from build123d import *

# Parameters (mm, degrees)
SKETCH1_W           = 279.4
SKETCH1_H           = 254
BOSS_EXTRUDE1_DEPTH = 4.800000052
SKETCH4_W           = 13.148347957
SKETCH4_H           = 12.442555781
SKETCH4_W_2         = 3.81
SKETCH4_H_2         = 12.7
SKETCH4_W_3         = 12.512633495
CUT_EXTRUDE1_DEPTH  = 378.628653575
FILLET1_R           = 6.35


with BuildPart() as part:
    # Sketch1 → Boss-Extrude1 (new body)
    with BuildSketch(Plane.XY):
        with Locations((139.7, 127)):
            Rectangle(SKETCH1_W, SKETCH1_H)
    extrude(amount=BOSS_EXTRUDE1_DEPTH)

    # Sketch4 → Cut-Extrude1 (cut, through all)
    with BuildSketch(Plane(origin=(0, 0, 0), x_dir=(-1, 0, 0), z_dir=(0, 0, -1))):
        Polygon((0, 0), (0, 72.724077305), (-18.411229684, 72.724077305), (-88.95741747, 143.27026509), (-105.001094941, 143.27026509), (-117.513728436, 143.27026509), (-161.28323771, 143.27026509), (-174.431585667, 143.27026509), (-190.55741747, 143.27026509), (-260.35, 73.47768256), (-279.4, 73.47768256), (-279.4, 0), align=None)
        Polygon((-190.5, 168.72768256), (-88.9, 168.72768256), (-50.8, 168.72768256), (0, 117.92768256), (0, 254), (-279.4, 254), (-279.4, 117.92768256), (-228.6, 168.72768256), align=None)
        with Locations((-167.857411689, 149.491542981)):
            Rectangle(SKETCH4_W, SKETCH4_H)
        with Locations((-139.75741747, 156.02768256)):
            Rectangle(SKETCH4_W_2, SKETCH4_H_2)
        with Locations((-111.257411689, 149.491542981)):
            Rectangle(SKETCH4_W_3, SKETCH4_H)
    extrude(amount=-CUT_EXTRUDE1_DEPTH, mode=Mode.SUBTRACT)

    # Fillet1
    fillet1_edges = [part.edges().sort_by_distance(p)[0] for p in [
        (18.411229684, 72.724077305, 2.400000026),
        (0, 72.724077305, 2.400000026),
        (279.4, 73.47768256, 2.400000026),
        (260.35, 73.47768256, 2.400000026),
        (174.431585667, 143.27026509, 2.400000026),
        (161.28323771, 143.27026509, 2.400000026),
        (117.513728436, 143.27026509, 2.400000026),
        (105.001094941, 143.27026509, 2.400000026),
        (228.6, 168.72768256, 2.400000026),
        (279.4, 117.92768256, 2.400000026),
        (0, 117.92768256, 2.400000026),
        (50.8, 168.72768256, 2.400000026),
    ]]
    fillet(fillet1_edges, radius=FILLET1_R)


solid = part.part
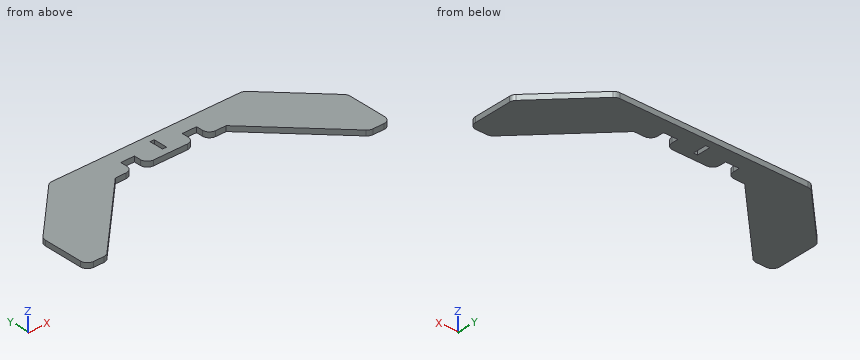
Verification items for the finished model (mm, model axes). Coordinates: 2 decimals unless noted, no trailing zeros. Write each loop counter-clockwise with the first axis right and the second up, starting at its lowest first coordinate (ties: lowest second). Pieces come first, ordered by that corner, then holes. Notation, with made-up numbers: (2, -30.5) -> (54, -30.5) arc R27 cw to (54, -6.5) -> close; hole circle Ø7 at (9, 10). An arc over 180 degrees is marked (long way). One line per item, written item: value. Start each with the question number.
Q1. Cross-section at B-B on y = 100.5. Enter the section's corners in (x, z).
Q2. Cross-section at C-C on x = 127. Enter the section's corners in (y, z), and give its area (3 significant figures).
Q3. Thickness scan on L1, parallel to X at y = 126.5, z = 2.8; L2, parallel to Y at x = 127, z = 4.1; L3, parallel to X at y = 110.5, z = 3.6. Record the ranges inside material, lowest first. Write a range as from..to.
Q4. Go/stop test with flat-tipped pins: P1, Ø1.4, axis at x = 165.5, z = 3, coming from the -Y side; P2, Ø1.9, axis at x = 140, z = 3, coming from the -Y side. Record where each tip stops, or that it passes through.
Q5. Cross-section at D-D on y = 138. Enter the section's corners in (x, z).
Checked values:
1. outline: (0, 0) -> (46.19, 0) -> (46.19, 4.8) -> (0, 4.8) -> close; (233.33, 0) -> (279.4, 0) -> (279.4, 4.8) -> (233.33, 4.8) -> close
2. outline: (143.27, 0) -> (168.73, 0) -> (168.73, 4.8) -> (143.27, 4.8) -> close
2. area: 122 mm²
3. L1: x = 8.57..72.19, 207.33..270.83
3. L2: y = 143.27..168.73
3. L3: x = 0..56.19, 223.33..279.4
4. P1: stops at y = 155.71
4. P2: stops at y = 143.27
5. outline: (20.07, 0) -> (83.69, 0) -> (83.69, 4.8) -> (20.07, 4.8) -> close; (195.83, 0) -> (259.33, 0) -> (259.33, 4.8) -> (195.83, 4.8) -> close
